Could you check a few things on this model? Use its own coordinates, in mm. Face numbers are marked on the shaded views. A direction names the side the tool comes from. Coordinates: 2 decimals unless noted, no trailing zeros. Loops run counter-clockwise (first coordinate to the right, second up) from the corner with the lowest first, then second, coordinate; pieces in that order, holes last. Notation, with made-up numbers: (87, 28) -> (121, 28) arc R13 cw to (121, 37) -> close; hole circle Ø8 at (0.5, -36.75). An arc over 180 degrees is marked (long way). One line per question, with ' | ' between items. Start each with the question number.
(1) Suppose I cut it at A-A (y = 7). Please give me the cut outline in (x, z), plus the area to 3 significant figures.
(2) Suppose I cut it at D-D (z = 2). Please give me the cut outline in (x, y), plus the area to 3 significant figures.
(3) If I drill on line 1 along X through (y, z) = (-15, -12); line 2 along X through (y, z) = (2.5, -13), over which ranges is the centre line in solid material (lowest first)?
(4) Which directions (+Z, -Z, +X, -X, +Y, -Y) give clear straight access to the entire face, cutting with the end or side of a thin tool? Please do the marked faces 1, 2, 3, 4 and 5.
(5) If we mould it in two halves opening along Z, with no side actions, what happens to the marked faces 6, 7, 8 and 9? For each: pulls with the +Z half, pulls with the -Z half, needs draft (parallel to the pull), parting line crosses it, or undercut.
(6) I'm going to push flat-ended pins straight in: pin 1 Ø22 at (x, z) = (9.5, 2.5) entering from -Y; pin 2 Ø4.5 at (y, z) = (10, -4) entering from -X; pin 3 Ø6 at (x, z) = (-19, -11) entering from +Y. Where does each tip first touch, or does it pass through?
(7) Suppose I cut it at B-B (x = 11). Please give me the cut outline in (y, z).
(8) Suppose I cut it at C-C (y = -12). Please give me the cut outline in (x, z), plus the area to 3 significant figures.
```python
from build123d import *

# Parameters (mm, degrees)
SKETCH_1_W                  = 50
SKETCH_1_H                  = 50
EXTRUDE_1_DEPTH             = 2
SKETCH_2_W                  = 3
SKETCH_2_H                  = 50
EXTRUDE_2_DEPTH             = 15
EXTRUDE_3_DEPTH             = 25
EXTRUDE_3_DEPTH_BACK        = 25
EXTRUDE_4_REACH             = 50.587
EXTRUDE_4_DIRECTION_2_REACH = 50.587
SKETCH_7_W                  = 93.751420651
SKETCH_7_H                  = 87.806812737
SKETCH_7_W_2                = 50
SKETCH_7_H_2                = 50
CUT_EXTRUDE_1_DEPTH         = 25
SKETCH_8_W                  = 44
SKETCH_8_H                  = 44
CUT_EXTRUDE_2_DEPTH         = 18
CHAMFER_1_SIZE              = 2


with BuildPart() as part:
    # 草图1 → 凸台-拉伸1 (new body)
    with BuildSketch(Plane(origin=(0, 0, 0), x_dir=(1, 0, 0), z_dir=(0, 1, 0))):
        Rectangle(SKETCH_1_W, SKETCH_1_H)
    extrude(amount=EXTRUDE_1_DEPTH)

    # 草图2 → 凸台-拉伸2 (add)
    with BuildSketch(Plane(origin=(0, 2, 0), x_dir=(1, 0, 0), z_dir=(0, 1, 0))):
        with Locations((-11.5, 0)):
            Rectangle(SKETCH_2_W, SKETCH_2_H)
        with Locations((11.5, 0)):
            Rectangle(SKETCH_2_W, SKETCH_2_H)
    extrude(amount=EXTRUDE_2_DEPTH)

    # 草图5 → 凸台-拉伸3 (add, two sides: drawn at the far end of the back side and taken through both)
    with BuildSketch(Plane(origin=(0, 0, 0), x_dir=(0, 0, -1), z_dir=(1, 0, 0)).offset(-EXTRUDE_3_DEPTH_BACK)):
        Polygon((25, 0), (0, 0), (0, -20), (36.547005384, -20), align=None)
        Polygon((0, 0), (-25, 0), (-36.547005384, -20), (0, -20), align=None)
    extrude(amount=EXTRUDE_3_DEPTH + EXTRUDE_3_DEPTH_BACK)

    # 凸台-拉伸4: up to this plane
    extrude_4_end = Plane(origin=(-25, 10.825317547, 18.75), z_dir=(0, 0.4999999999999978, 0.86602540378444))
    # 草图6 → 凸台-拉伸4 (add, up to the surface)
    with BuildSketch(Plane.XY, mode=Mode.PRIVATE) as extrude_4_sk1:
        Polygon((-25, 0), (-36.547005384, -20), (-25, -20), align=None)
    extrude_4_tool1 = split(extrude(extrude_4_sk1.sketch, amount=EXTRUDE_4_REACH, mode=Mode.PRIVATE), bisect_by=extrude_4_end, keep=Keep.BOTH, mode=Mode.PRIVATE)
    extrude_4 = extrude_4_tool1.solids().sort_by_distance((-28.849002, -13.333333, 0))[0]
    add(extrude_4)

    # 凸台-拉伸4 direction 2: up to this plane
    extrude_4_direction_2_end = Plane(origin=(-25, 10.825317547, -18.75), z_dir=(0, -0.4999999999999978, 0.86602540378444))
    # 草图6 → 凸台-拉伸4 direction 2 (add, up to the surface)
    with BuildSketch(Plane.XY, mode=Mode.PRIVATE) as extrude_4_direction_2_sk1:
        Polygon((-25, 0), (-36.547005384, -20), (-25, -20), align=None)
    extrude_4_direction_2_tool1 = split(extrude(extrude_4_direction_2_sk1.sketch, amount=-EXTRUDE_4_DIRECTION_2_REACH, mode=Mode.PRIVATE), bisect_by=extrude_4_direction_2_end, keep=Keep.BOTH, mode=Mode.PRIVATE)
    extrude_4_direction_2 = extrude_4_direction_2_tool1.solids().sort_by_distance((-28.849002, -13.333333, 0))[0]
    add(extrude_4_direction_2)
    extrude_4 = extrude_4 + extrude_4_direction_2  # both directions under the feature's name, for the pattern or mirror that repeats it

    # 镜向1: 凸台-拉伸4 across plane
    add(extrude_4.mirror(Plane(origin=(0, 0, 0), x_dir=(0, 0, 1), z_dir=(1, 0, 0))))

    # 草图7 → 切除-拉伸1 (cut)
    with BuildSketch(Plane(origin=(0, 2, 0), x_dir=(1, 0, 0), z_dir=(0, 1, 0))):
        with Locations((6.640722021, -2.029388647)):
            Rectangle(SKETCH_7_W, SKETCH_7_H)
        Rectangle(SKETCH_7_W_2, SKETCH_7_H_2, mode=Mode.SUBTRACT)
    extrude(amount=-CUT_EXTRUDE_1_DEPTH, mode=Mode.SUBTRACT)

    # 草图8 → 切除-拉伸2 (cut)
    with BuildSketch(Plane.XZ.offset(20)):
        Rectangle(SKETCH_8_W, SKETCH_8_H)
    extrude(amount=-CUT_EXTRUDE_2_DEPTH, mode=Mode.SUBTRACT)

    # 倒角1
    chamfer_1_edges = [part.edges().sort_by_distance(p)[0] for p in [
        (-22, -20, 0),
        (0, -20, -22),
        (22, -20, 0),
        (0, -20, 22),
    ]]
    chamfer(chamfer_1_edges, length=CHAMFER_1_SIZE)


solid = part.part
```
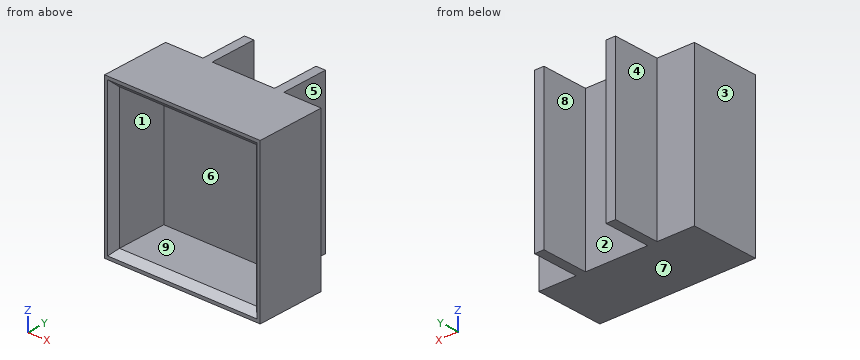
Checks:
1) outline: (-13, -25) -> (-10, -25) -> (-10, 25) -> (-13, 25) -> close; (10, -25) -> (13, -25) -> (13, 25) -> (10, 25) -> close | area: 300 mm^2
2) outline: (-25, -20) -> (-24, -20) -> (-22, -18) -> (-22, -2) -> (22, -2) -> (22, -18) -> (24, -20) -> (25, -20) -> (25, 2) -> (13, 2) -> (13, 17) -> (10, 17) -> (10, 2) -> (-10, 2) -> (-10, 17) -> (-13, 17) -> (-13, 2) -> (-25, 2) -> close | area: 394 mm^2
3) line 1: x = -25 to -22, 22 to 25 | line 2: x = -13 to -10, 10 to 13
4) face 1: -Y | face 2: +Z, -Z, +Y | face 3: +Z, -Z, -X, +Y, -Y | face 4: +Z, -Z, -X, +Y | face 5: +Z, -Z, +X, +Y
5) face 6: undercut | face 7: pulls with the -Z half | face 8: needs draft | face 9: undercut
6) pin 1: stops at y = -2 | pin 2: stops at x = -13 | pin 3: stops at y = 2
7) outline: (-20, -25) -> (17, -25) -> (17, 25) -> (-20, 25) -> (-20, 24) -> (-18, 22) -> (-2, 22) -> (-2, -22) -> (-18, -22) -> (-20, -24) -> close
8) outline: (-25, -25) -> (25, -25) -> (25, 25) -> (-25, 25) -> close; hole (-22, -22) -> (22, -22) -> (22, 22) -> (-22, 22) -> close | area: 564 mm^2
